Design review of the part shown in the three views and the two pictorial views. Dimensions are in mm from the part's minimum x, y and z. Give positions to 0.01 mm unless a question says otherwise; leave off trailing zeros. Order: outer loops, then holes, each group sorted by start corner. A loop starts at its lowest first (then second) coordinate and runs counter-clockwise, first axis right, second up. Notation, with made-up numbers: M 22,-5.75 L 56,-5.75 A32 ccw 56,26.25 Z; hole C 71,-18 d4. An arc over 180 degrees is marked long. Answer as a JSON object with one key per item and string values.
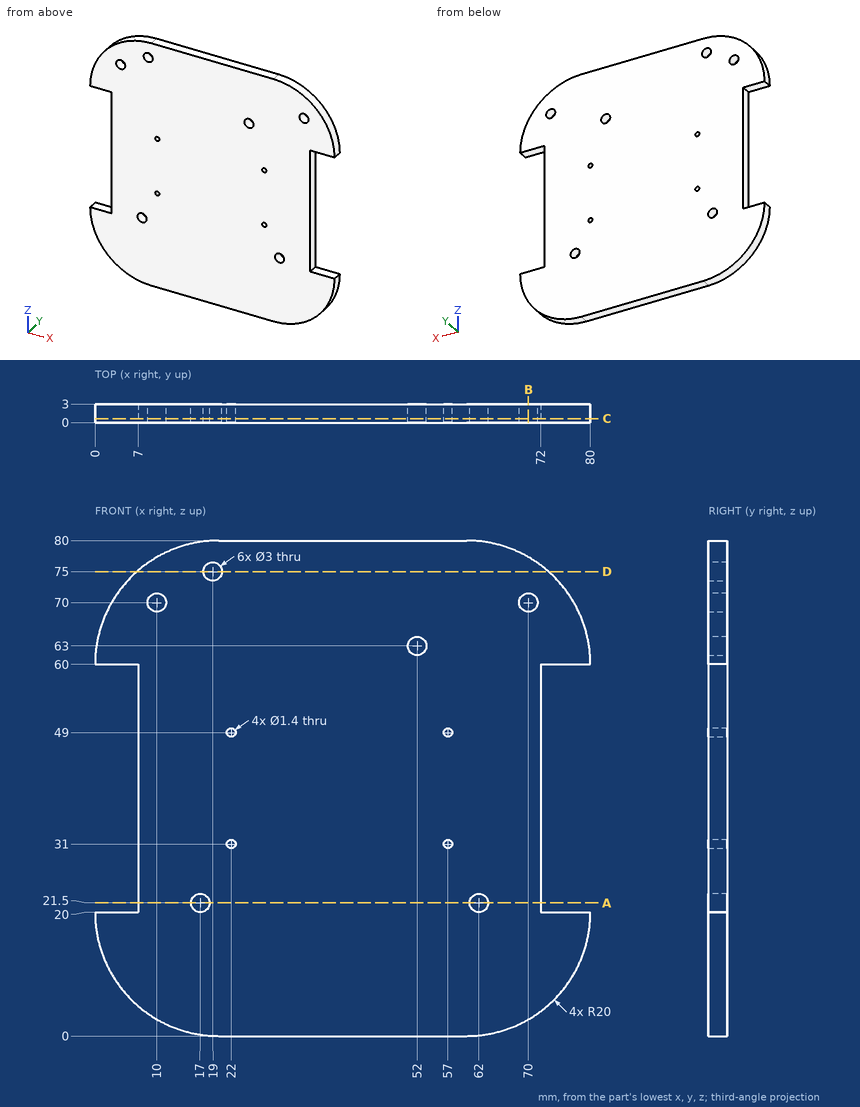
(1) To check wall thickness, follow L1, parallel to X at y = 2.5, z = 31; L2, parallel to X at y = 0.65, z = 70; L3, parallel to Z at x = 18, y = 1.45. State the ranges of each line that lie inside material, in increasing order. Write a range as from..to.
Checked values:
{"L1": "x = 7..21.3, 22.7..56.3, 57.7..72", "L2": "x = 2.68..8.5, 11.5..68.5, 71.5..77.32", "L3": "z = 0.1..20.38, 22.62..73.88, 76.12..79.9"}
(2) Insertion check: pin 1 (1.5 mm diameter, centred on x = 77, y = 1, fed in from +Z); pin 2 (0.9 mm diameter, centred on y = 1.5, z = 38, fed in from -X); pin 3 (1.3 mm diameter, centred on x = 22, z = 31, fed in from -Y); pin 4 (1 mm diameter, centred on y = 2, z = 38.5, fed in from +X). Each pin has a flat end and moves straight along its axis. Give the tip position at first contact, or say it passes through.
Checked values:
{"pin 1": "stops at z = 71.66", "pin 2": "stops at x = 7", "pin 3": "passes through", "pin 4": "stops at x = 72"}
(3) We need section B-B (x = 70). Write out the cut boundary in (y, z).
Checked values:
{"outline": "M 0,2.68 L 3,2.68 L 3,68.5 L 0,68.5 Z; M 0,71.5 L 3,71.5 L 3,77.32 L 0,77.32 Z"}
(4) We need section C-C (y = 0.65). Count the separate pieces of the cut face and the enclosed holes in it, plus the area to 3 significant figures.
Checked values:
{"separate pieces": "1", "enclosed holes": "10", "area": "5,410 mm^2"}
(5) We need section A-A (z = 21.5). Write out the cut boundary in (x, y), plus the area to 3 significant figures.
Checked values:
{"outline": "M 7,0 L 15.5,0 L 15.5,3 L 7,3 Z; M 18.5,0 L 60.5,0 L 60.5,3 L 18.5,3 Z; M 63.5,0 L 72,0 L 72,3 L 63.5,3 Z", "area": "177 mm^2"}
(6) We need section D-D (z = 75). Write out the cut boundary in (x, y).
Checked values:
{"outline": "M 6.77,0 L 17.5,0 L 17.5,3 L 6.77,3 Z; M 20.5,0 L 73.23,0 L 73.23,3 L 20.5,3 Z"}
